Geometry: final body of the model. Coordinates: model frame, mm. Face numbers are marked on the shaded views. A direction names the side the tool comes from. Give positions to 0.01 mm unless a question says otherwise; leave off trailing zeros. Write each loop counter-clockwise with the first axis right and the second up, starting at its lowest first coordinate (ties: lowest second). Pieces come first, ordered by that corner, then holes. Notation, with made-up numbers: M -14.75,3 L -7.75,3 A13 cw -7.75,12 Z; hole C -30,61 d6. An arc over 180 degrees is marked long. Use a Markdown table: item, result. Add a question column.
1) Line query: line 1 (X direction, y = -12, z = 27); line 2 (Y direction, x = 4, z = 8); line 3 (Z direction, x = 33, y = -8.5). Output: solid intervals per line, ascending.
2) Pin query (flat end, axial travel): pin 1 (9.5 mm diameter, centred on y = -9, z = 31.5, fed in from +X); pin 2 (9.5 mm diameter, centred on x = 33, y = -11, fed in from +Z); pin 3 (9.5 mm diameter, centred on x = 12.5, y = 6.5, fed in from +Z). Return the tip coordinate at first contact, or that it passes through.
3) Section A-A on x = 26.5. Return the cut outline in (y, z).
4) Set-up query: the marked faces 1, 2 and 3. Return all of +Z, -Z, +X, -X, +Y, -Y with unobstructed straight access to the full face (end or side cutting, diameter ignored); none if empty.
5) Section D-D on y = 11.5. Return the cut outline in (x, z).
6) Section B-B on y = -16. Return the cut outline in (x, z), then the cut area to 3 significant figures.
7) Section C-C on z = 34.5. Return the cut outline in (x, y).
```python
from build123d import *

# Parameters (mm, degrees)
F0_W      = 19.05
F0_H      = 19.05
F1_DEPTH  = 19.05
F2_W      = 19.05
F2_H      = 19.05
F3_DEPTH  = 19.05
F3_FACE_W = 19.05
F3_FACE_H = 19.05
F4_DEPTH  = 19.05


with BuildPart() as f1:
    # F0 (on Front) → F1 (new body)
    with BuildSketch(Plane.XZ):
        with Locations((9.525, 9.525)):
            Rectangle(F0_W, F0_H)
        with Locations((9.525, -9.525)):
            Rectangle(F0_W, F0_H)
        with Locations((28.575, -9.525)):
            Rectangle(F0_W, F0_H)
        with Locations((28.575, 9.525)):
            Rectangle(F0_W, F0_H)
        with Locations((9.525, 28.575)):
            Rectangle(F0_W, F0_H)
    extrude(amount=F1_DEPTH)

    # F2 (on Front) → F3 (join)
    with BuildSketch(Plane.XZ):
        with Locations((9.525, -9.525)):
            Rectangle(F2_W, F2_H)
    extrude(amount=-F3_DEPTH)

    # F3_face (on face) → F4 (join)
    with BuildSketch(Plane(origin=(19.05, 9.525, -9.525), x_dir=(0, 1, 0), z_dir=(1, 0, 0))):
        Rectangle(F3_FACE_W, F3_FACE_H)
    extrude(amount=F4_DEPTH)


solid = f1.part
```
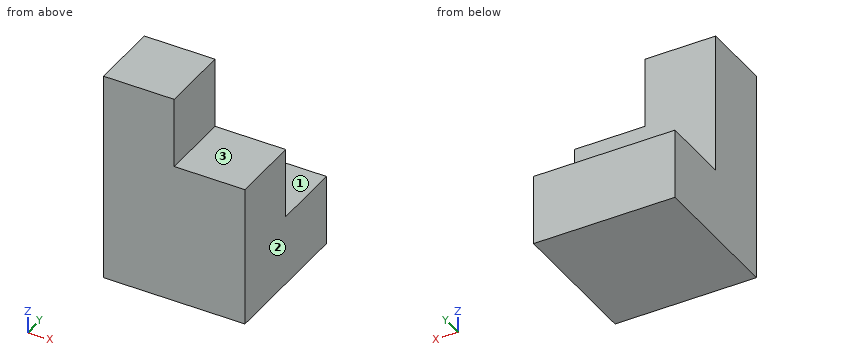
Found:
| question | item | result |
|---|---|---|
| 1 | line 1 | 0 to 19.05 |
| 1 | line 2 | -19.05 to 0 |
| 1 | line 3 | -19.05 to 19.05 |
| 2 | pin 1 | x = 19.05 |
| 2 | pin 2 | z = 19.05 |
| 2 | pin 3 | z = 0 |
| 3 | outline | M -19.05,-19.05 L 19.05,-19.05 L 19.05,0 L 0,0 L 0,19.05 L -19.05,19.05 Z |
| 4 | face 1 | +Z, +X, -X, +Y |
| 4 | face 2 | +Z, -Z, +X, +Y, -Y |
| 4 | face 3 | +Z, +X, +Y, -Y |
| 5 | outline | M 0,-19.05 L 38.1,-19.05 L 38.1,0 L 0,0 Z |
| 6 | outline | M 0,-19.05 L 38.1,-19.05 L 38.1,19.05 L 19.05,19.05 L 19.05,38.1 L 0,38.1 Z |
| 6 | area | 1,810 mm² |
| 7 | outline | M 0,-19.05 L 19.05,-19.05 L 19.05,0 L 0,0 Z |
